Check sheet for the modelled part. Datum: model origin and axes. Units: mm. Face numbers are marked on the shaded views. A direction names the side the tool comes from. Round coordinates to 2 decimals unless told otherwise and drop trailing zeros. Write each loop counter-clockwise with the first axis right and the second up, starting at its lowest first coordinate (ties: lowest second). Pieces come first, ordered by that corner, then holes. Notation, with made-up numbers: M 36,89.5 L 54,89.5 A13 ccw 54,94.5 Z; hole C -16.5,-39 d3. An arc over 180 degrees is marked long. Put each result on its own line as item: value.
```python
from build123d import *

# Parameters (mm, degrees)
SKETCH1_R                       = 41.275
BOSS_EXTRUDE1_DEPTH             = 25.4
SKETCH2_OUTSIDE_W               = 108.444
SKETCH2_OUTSIDE_H               = 108.444
SKETCH2_OUTSIDE_R               = 22.225
CUT_EXTRUDE1_DEPTH              = 19.05
SKETCH3_R                       = 15.875
CUT_EXTRUDE2_DEPTH              = 26.4
F_4_40_TAPPED_HOLE1_D           = 2.2606
F_4_40_TAPPED_HOLE1_DEPTH       = 7.5946
F_4_40_TAPPED_HOLE1_TIP         = 0.679152758
F_5_32_0_15625_DIAMETER_HOLE1_D = 3.96875
MIRROR2_COPY_1_D                = 3.96875
MIRROR2_COPY_2_D                = 3.96875


with BuildPart() as part:
    # Sketch1 → Boss-Extrude1 (new body)
    with BuildSketch(Plane.XY):
        Circle(SKETCH1_R)
    extrude(amount=BOSS_EXTRUDE1_DEPTH)

    # Sketch2 outside → Cut-Extrude1 (cut)
    with BuildSketch(Plane(origin=(0, 0, 0), x_dir=(-1, 0, 0), z_dir=(0, 0, -1))):
        Rectangle(SKETCH2_OUTSIDE_W, SKETCH2_OUTSIDE_H)
        Circle(SKETCH2_OUTSIDE_R, mode=Mode.SUBTRACT)
    extrude(amount=-CUT_EXTRUDE1_DEPTH, mode=Mode.SUBTRACT)

    # Sketch3 → Cut-Extrude2 (cut, through all)
    with BuildSketch(Plane(origin=(0, 0, 0), x_dir=(-1, 0, 0), z_dir=(0, 0, -1))):
        Circle(SKETCH3_R)
    extrude(amount=-CUT_EXTRUDE2_DEPTH, mode=Mode.SUBTRACT)

    # #4-40 Tapped Hole1
    with Locations(Plane(origin=(0, 0, 0), x_dir=(-1, 0, 0), z_dir=(0, 0, -1))):
        with Locations((0, 18.415), (0, -18.415)):
            Hole(F_4_40_TAPPED_HOLE1_D / 2, depth=F_4_40_TAPPED_HOLE1_DEPTH)
            with Locations((0, 0, -(F_4_40_TAPPED_HOLE1_DEPTH + F_4_40_TAPPED_HOLE1_TIP / 2))):  # 118° drill point
                Cone(0, F_4_40_TAPPED_HOLE1_D / 2, F_4_40_TAPPED_HOLE1_TIP, mode=Mode.SUBTRACT)

    # 5/32 (0.15625) Diameter Hole1 (through all)
    with Locations(Plane.XY.offset(25.4)):
        with Locations((0, 38.1), (38.1, 0)):
            f_5_32_0_15625_diameter_hole1 = Hole(F_5_32_0_15625_DIAMETER_HOLE1_D / 2)

    # Mirror1: 5/32 (0.15625) Diameter Hole1 across plane
    add(f_5_32_0_15625_diameter_hole1.mirror(Plane.ZX), mode=Mode.SUBTRACT)

    # Mirror2 copy 1 (through all)
    with Locations(Plane(origin=(0, 0, 25.4), x_dir=(-1, 0, 0), z_dir=(0, 0, 1))):
        with Locations((0, 38.1), (38.1, 0)):
            Hole(MIRROR2_COPY_1_D / 2)

    # Mirror2 copy 2 (through all)
    with Locations(Plane(origin=(0, 0, 25.4), x_dir=(-1, 0, 0), z_dir=(0, 0, 1))):
        with Locations((0, -38.1), (38.1, 0)):
            Hole(MIRROR2_COPY_2_D / 2)


solid = part.part
```
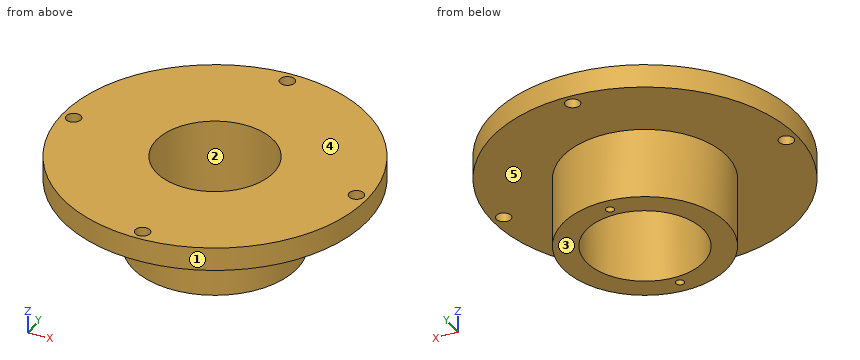
1. Scan lines: probe 1 along Y at (x, z) = (0, 23.5) (3 decimals); probe 2 along Y at (x, z) = (0, 4.25) (3 decimals); probe 3 along Y at (x, z) = (38.1, 22.25) (3 decimals). Record each from-to range of solid material in increasing order.
Computed values:
probe 1: y = -41.275 to -40.084, -36.116 to -15.875, 15.875 to 36.116, 40.084 to 41.275
probe 2: y = -22.225 to -19.545, -17.285 to -15.875, 15.875 to 17.285, 19.545 to 22.225
probe 3: y = -15.875 to -1.984, 1.984 to 15.875
2. Access from +Z, -Z, +X, -X, +Y, -Y to the whole of each face (thin tool, end or side, straight path). Record for the marked faces 4 and 5.
Computed values:
face 4: +Z, +X, -X, +Y, -Y
face 5: -Z
3. Depth check by flat-ended pin: pin 1 Ø5 at (x, y) = (0, -38.1) entering from -Z; pin 2 Ø4 at (y, z) = (1, 17) entering from -X (3 decimals). Enter the tip coordinate at first touch or a pass-through.
Computed values:
pin 1: stops at z = 19.05
pin 2: stops at x = -22.225
4. Cross-section at A-A (x = 38.1). Enter the section's corners in (y, z) (3 decimals), then the cut area to 3 significant figures.
Computed values:
outline: M -15.875,19.05 L -1.984,19.05 L -1.984,25.4 L -15.875,25.4 Z; M 1.984,19.05 L 15.875,19.05 L 15.875,25.4 L 1.984,25.4 Z
area: 176 mm2
5. Cross-section at B-B (y = 0). Enter the section's corners in (x, z) (3 decimals).
Computed values:
outline: M -41.275,19.05 L -40.084,19.05 L -40.084,25.4 L -41.275,25.4 Z; M -36.116,19.05 L -22.225,19.05 L -22.225,0 L -15.875,0 L -15.875,25.4 L -36.116,25.4 Z; M 15.875,0 L 22.225,0 L 22.225,19.05 L 36.116,19.05 L 36.116,25.4 L 15.875,25.4 Z; M 40.084,19.05 L 41.275,19.05 L 41.275,25.4 L 40.084,25.4 Z
6. Release check for a two-part mould opening along X. For the marked faces 1, 2 and 3 record: +X half, -X half, draft (parallel to the pull), parting line (faces both ways), or undercut.
Computed values:
face 1: parting line
face 2: undercut
face 3: draft
7. Cross-section at D-D (z = 13). Enter the section's corners in (x, y) (3 decimals).
Computed values:
outline: C 0,0 d44.45; hole C 0,0 d31.75
